Could you check a few things on this model? Use its own coordinates, in mm. Coordinates: 2 decimals unless noted, no trailing zeros. Order: outer loops, then holes, each group sorted by start corner. A loop starts at its lowest first (then second) coordinate and runs counter-clockwise, first axis right, second up. Notation, with made-up numbers: (49, -31) -> (70, -31) arc R8 ccw to (70, -27) -> close; hole circle Ø9 at (47, 31.5). An arc over 180 degrees is marked (long way). Put each result on its own line as item: value. Start each with the question number.
Q1. Please list where these lines run through material, in increasing order: line 1 along Y through (x, z) = (0, 0.5) (3 decimals); line 2 along X through (y, z) = (0, 0.35); line 3 along X through (y, z) = (0.75, 0.5).
Q2. If we section it at A-A (x = 0): Please give me the cut outline in (y, z) (3 decimals), and give its area (3 significant figures).
Q3. We'd pull the mould along Y, two halves only. Please class faces 1 (the face through (-0.434, 1.952, 0.37)), 2 (the face through (-0.1, 2.3, 0.75)): +Y half, -Y half, draft (parallel to the pull), parting line (faces both ways), or undercut.
Q4. If we section it at C-C (z = 0.6): Please give me the cut outline in (x, y) (3 decimals), and give its area (3 significant figures).
Q5. If we section it at B-B (y = 0): Please give me the cut outline in (x, z).
Autodesk Inventor part; units mm, degrees
ref_plane "YZ Plane" through (0, 0, 0) normal (1, 0, 0) x (0, 1, 0)
ref_plane "XZ Plane" through (0, 0, 0) normal (0, 1, 0) x (-1, 0, 0)
ref_plane "XY Plane" through (0, 0, 0) normal (0, 0, 1) x (1, 0, 0)
sketch "Sketch1" plane through (0, 0, 0) normal (0, 0, 1) x (1, 0, 0)
  circle A0 centre (0, 0) radius 2
  line L0 (0, 0) -> (7.366, 0)
  line L1 (0, 0) -> (-7.366, 0)
  line L2 (7.366, 0) -> (7.366, 9.525)
  line L3 (-7.366, 0) -> (-7.366, -9.525)
  line L4 (-7.366, -9.525) -> (7.366, -9.525)
  line L5 (7.366, -9.525) -> (7.366, 9.525)
  line L6 (7.366, 9.525) -> (-7.366, 9.525)
  line L7 (-7.366, 9.525) -> (-7.366, -9.525)
  point P0 (7.366, 0)
  dimension "d0" = 4
  dimension "d1" = 7.366
  dimension "d2" = 7.366
  dimension "d3" = 9.525
  dimension "d4" = 9.525
extrude "Extrusion1" add sketch "Sketch1" along normal blind 0.75 contours L0 L5 L4 L3 L1 A0 | A0 L1 L7 L6 L2 L0
equation "\"d2\" = d1"
equation "\"d4\" = d3"
properties part number "MotorProtector"
The answers:
1. line 1: -9.525 to -2, 2 to 9.525
1. line 2: -7.37 to -2, 2 to 7.37
1. line 3: -7.37 to -1.85, 1.85 to 7.37
2. outline: (-9.525, 0) -> (-2, 0) -> (-2, 0.75) -> (-9.525, 0.75) -> close; (2, 0) -> (9.525, 0) -> (9.525, 0.75) -> (2, 0.75) -> close
2. area: 11.3 mm^2
3. face 1: undercut
3. face 2: draft
4. outline: (-7.366, -9.525) -> (7.366, -9.525) -> (7.366, 9.525) -> (-7.366, 9.525) -> close; hole circle Ø4 at (0, 0)
4. area: 268 mm^2
5. outline: (-7.37, 0) -> (-2, 0) -> (-2, 0.75) -> (-7.37, 0.75) -> close; (2, 0) -> (7.37, 0) -> (7.37, 0.75) -> (2, 0.75) -> close
